The figure shows three views and two pictorial views of one solid part (mm, origin at its lowest corner). Answer the questions. Round coordinates to 2 decimals unless told otherwise and drop trailing zeros. Order: outer loops, then holes, each group sorted by start corner. A loop starts at its lowest first (then second) coordinate and runs counter-clockwise, first axis right, second up. Notation, with made-up numbers: (-36.5, -18.5) - (-10.5, -18.5) arc R12 cw to (-10.5, -7.5) - close; hole circle Ø1 at (-26.75, 78.25). An arc over 180 degrees is marked (long way). Use CSV: the item, a comma, the result in double quotes. Start each with the question number.
Item 1: Straight lines are drawn through the part: line 1 along Y through (x, z) = (5, 5); line 2 along Y through (x, z) = (3.5, 24.25); line 3 along Z through (x, y) = (4.5, 25.75). For each, find the intervals that lie inside material, in ascending order. Write a range as [from, to].
Item 2: Determine the mould class of the marked faces 1, 2 and 3 for opening direction Z: +Z half, -Z half, draft (parallel to the pull), parting line (faces both ways), or undercut.
Item 3: Find section B-B, the plane x = 0.75. Give the vertices of the cut face in (y, z), plus the area to 3 significant figures.
Item 4: Find section A-A, the plane y = 15. Give the vertices of the cut face in (x, z).
Item 5: Flat-ended cylindrical pins translate along their axes: P1, Ø3.5, axis at y = 25, z = 5, coming from the +X side; P2, Ø5, axis at y = 5, z = 5, coming from the +X side. Find the tip coordinate at first contact, or state that the pin passes through.
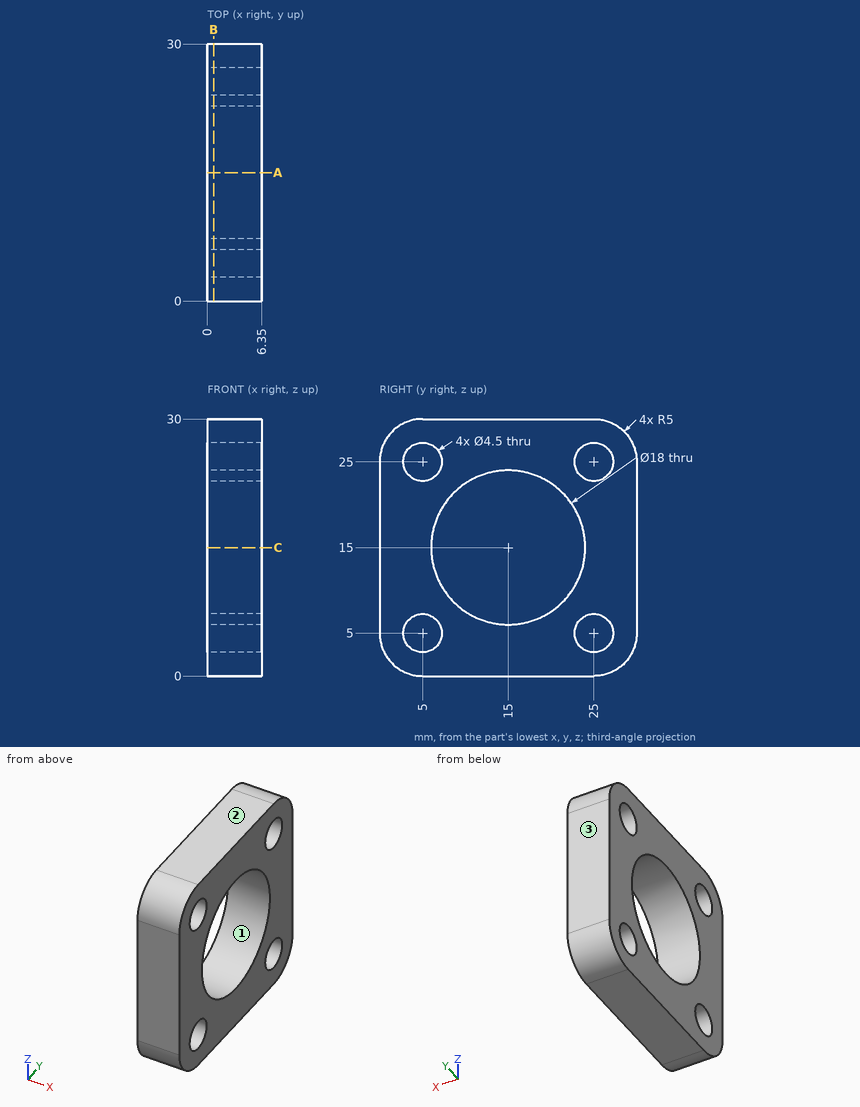
Worked out:
1,line 1,"y = [0, 2.75], [7.25, 22.75], [27.25, 30]"
1,line 2,"y = [0, 2.88], [7.12, 22.88], [27.12, 30]"
1,line 3,"z = [0.06, 2.88], [7.12, 22.88], [27.12, 29.94]"
2,face 1,"undercut"
2,face 2,"+Z half"
2,face 3,"draft"
3,outline,"(0, 5) arc R5 ccw to (5, 0) - (25, 0) arc R5 ccw to (30, 5) - (30, 25) arc R5 ccw to (25, 30) - (5, 30) arc R5 ccw to (0, 25) - close; hole circle Ø4.5 at (5, 5); hole circle Ø4.5 at (5, 25); hole circle Ø18 at (15, 15); hole circle Ø4.5 at (25, 5); hole circle Ø4.5 at (25, 25)"
3,area,"560 mm²"
4,outline,"(0, 0) - (6.35, 0) - (6.35, 6) - (0, 6) - close; (0, 24) - (6.35, 24) - (6.35, 30) - (0, 30) - close"
5,P1,"passes through"
5,P2,"stops at x = 6.35"
